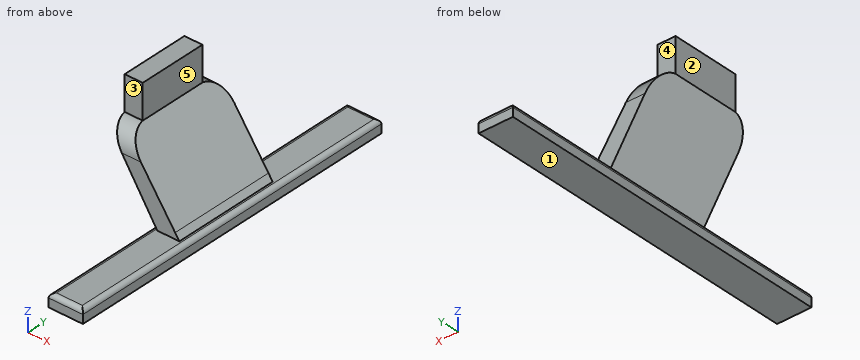
```python
from build123d import *

# Parameters (mm, degrees)
F0_W        = 4.2
F0_H        = 16
F1_DEPTH    = 8
F4_DEPTH    = 12.5
F5_W        = 8
F5_H        = 80
F6_DEPTH    = 3
F7_R        = 1
F8_T1_DEPTH = 29.0746859277


# Not quite as in the source:
# - a fillet or chamfer that OpenCascade refuses, or shapes differently, is made with other operations: its cross-section is extruded or revolved along the edge and cut away or added


with BuildPart() as f1:
    # F0 (on Top) → F1 (new body)
    with BuildSketch(Plane.XY):
        Rectangle(F0_W, F0_H)
    extrude(amount=F1_DEPTH)

    # F3 (on face) → F4 (join, symmetric)
    with BuildSketch(Plane.XZ):
        Polygon((13.571528727, -16.3830408858), (2.1, 0), (-0.9, 0), (11.558498512, -17.792579817), align=None)
        Polygon((14.558498512, -17.792579817), (13.571528727, -16.3830408858), (11.558498512, -17.792579817), align=None)
        Polygon((11.558498512, -17.792579817), (-0.9, 0), (-2.1, 0), (9.4175692648, -17.792579817), align=None)
    extrude(amount=F4_DEPTH, both=True)

    # F5 (on face) → F6 (join)
    with BuildSketch(Plane(origin=(0, 0, -17.792579817), x_dir=(1, 0, 0), z_dir=(0, 0, -1))):
        with Locations((11.9880338884, 0)):
            Rectangle(F5_W, F5_H)
    extrude(amount=F6_DEPTH)

    # F7
    f7_edges = [f1.edges().sort_by_distance(p)[0] for p in [
        (15.988034, 0, -17.79258),
        (11.988034, 40, -17.79258),
        (7.988034, 0, -17.79258),
        (11.988034, -40, -17.79258),
    ]]
    fillet(f7_edges, radius=F7_R)

    # F8: fillet of radius 5 on 2 edges, made by hand

    # F8_s2 → F8_t1 (cut)
    with BuildSketch(Plane.YZ.offset(-14.5373429638)):
        with BuildLine():
            ThreePointArc((-12.5, -4.9749371855), (-11.2080992435, -1.6208352193), (-8, 0))
            Line((-8, 0), (-12.5, 0))
            Line((-12.5, 0), (-12.5, -4.9749371855))
        make_face()
        with BuildLine():
            ThreePointArc((12.5, -4.9749371855), (11.2080992435, -1.6208352193), (8, 0))
            Line((8, 0), (12.5, 0))
            Line((12.5, 0), (12.5, -4.9749371855))
        make_face()
    extrude(amount=F8_T1_DEPTH, mode=Mode.SUBTRACT)


solid = f1.part
```
Geometry: final body of the model. Coordinates: model frame, mm. Face numbers are marked on the shaded views. A direction names the side the tool comes from. Give positions to 0.01 mm unless a question says otherwise; leave off trailing zeros. Loops run counter-clockwise (first coordinate to the right, second up) from the corner with the lowest first, then second, coordinate; pieces in that order, holes last. Notation, with made-up numbers: (54.5, -9.5) -> (104.5, -9.5) arc R19 cw to (104.5, -1.5) -> close; hole circle Ø8 at (79.5, -39). An arc over 180 degrees is marked (long way). Return JSON: item names as keys, results as strings.
Item 1: Pin query (flat end, axial travel): P1, Ø0.6, axis at y = -1.5, z = -20.5, coming from the -X side; P2, Ø4, axis at x = 5, y = -18, coming from the -Z side; P3, Ø4.5, axis at x = 1, z = 5, coming from the -Y side; P4, Ø10.5, axis at x = 5.5, z = -13, coming from the -Y side. Return the tip coordinate at first contact, or that it passes through.
Filled in:
{"P1": "x = 7.99", "P2": "through", "P3": "y = -8", "P4": "y = -12.5"}
Item 2: Section A-A, the plane y = -14.5. Output: boundary loops of the cut face in (x, z), plus the area to 3 significant figures.
Filled in:
{"outline": "(7.99, -20.79) -> (15.99, -20.79) -> (15.99, -18.79) arc R1 ccw to (14.99, -17.79) -> (8.99, -17.79) arc R1 ccw to (7.99, -18.79) -> close", "area": "23.6 mm^2"}
Item 3: Access query for the marked faces 1, 2, 3, 4 and 5. Directions: +Z, -Z, +X, -X, +Y, -Y. A direction counts if a zero-diameter tool reaches every point of the face in a straight line with its end or side. Return the directions, or none.
Filled in:
{"face 1": "-Z, +X, -X, +Y, -Y", "face 2": "+Z, -Z, -X, +Y, -Y", "face 3": "+Z, +X, -X, -Y", "face 4": "+Z, +X, -X, +Y", "face 5": "+Z, +X, +Y, -Y"}
Item 4: Section C-C, the plane x = 3.5. Output: boundary loops of the cut face in (y, z), plus the area to 3 significant figures.
Filled in:
{"outline": "(-12.5, -8.65) -> (12.5, -8.65) -> (12.5, -4.97) arc R5 ccw to (11.52, -2) -> (-11.52, -2) arc R5 ccw to (-12.5, -4.97) -> close", "area": "164 mm^2"}
Item 5: Line query: line 1 (Z direction, x = 13.75, y = -24); line 2 (Z direction, x = -0.75, y = 4); line 3 (Z direction, x = 8.25, y = -4.5). Output: solid intervals per line, ascending.
Filled in:
{"line 1": "-20.79 to -17.79", "line 2": "-2.09 to 8", "line 3": "-20.79 to -18.12, -15.99 to -8.78"}
Item 6: Section D-D, the plane z = -3. Output: boundary loops of the cut face in (x, y), plus the area to 3 significant figures.
Filled in:
{"outline": "(-0.16, -12.09) -> (4.2, -12.09) -> (4.2, 12.09) -> (-0.16, 12.09) -> close", "area": "105 mm^2"}
Item 7: Section B-B, the plane z = 6.25. Output: boundary loops of the cut face in (x, y), plus the area to 3 significant figures.
Filled in:
{"outline": "(-2.1, -8) -> (2.1, -8) -> (2.1, 8) -> (-2.1, 8) -> close", "area": "67.2 mm^2"}
